from build123d import *

# Parameters (mm, degrees)
SKETCH_1_W          = 200
SKETCH_1_H          = 100
EXTRUDE_1_DEPTH     = 8
SKETCH_2_OUTSIDE_W  = 246.75
SKETCH_2_OUTSIDE_H  = 146.75
CUT_EXTRUDE_1_DEPTH = 223.081848133
SKETCH_3_R          = 2
SKETCH_3_R_2        = 4
CUT_EXTRUDE_2_DEPTH = 184.742611471


with BuildPart() as part:
    # 草图1 → 凸台-拉伸1 (new body)
    with BuildSketch(Plane.XY):
        with Locations((100, 46.209912536)):
            Rectangle(SKETCH_1_W, SKETCH_1_H)
    extrude(amount=EXTRUDE_1_DEPTH)

    # 草图2 outside → 切除-拉伸1 (cut, through all)
    with BuildSketch(Plane.XY.offset(8)):
        with Locations((100, 46.21)):
            Rectangle(SKETCH_2_OUTSIDE_W, SKETCH_2_OUTSIDE_H)
        with BuildLine():
            Line((156, 96.209912536), (156, 53.259476571))
            ThreePointArc((156, 53.259476571), (97.731456144, 1.942362699), (44, 57.992340397))
            Line((44, 57.992340397), (44, 96.209912536))
            Line((44, 96.209912536), (56, 96.209912536))
            Line((56, 96.209912536), (56, 57.992340397))
            ThreePointArc((56, 57.992340397), (98, 13.942368774), (144, 53.797105004))
            Line((144, 53.797105004), (144, 96.209912536))
            Line((144, 96.209912536), (156, 96.209912536))
        make_face(mode=Mode.SUBTRACT)
    extrude(amount=-CUT_EXTRUDE_1_DEPTH, mode=Mode.SUBTRACT)

    # 草图3 → 切除-拉伸2 (cut, through all)
    with BuildSketch(Plane.XY.offset(13)):
        with Locations((48.3, 87.392340397)):
            Circle(SKETCH_3_R)
        with Locations((56.8, 35.392340397)):
            Circle(SKETCH_3_R)
        with Locations((143.2, 35.392340397)):
            Circle(SKETCH_3_R)
        with Locations((151.7, 87.392340397)):
            Circle(SKETCH_3_R)
        with Locations((100, 7.692340397)):
            Circle(SKETCH_3_R_2)
    extrude(amount=-CUT_EXTRUDE_2_DEPTH, mode=Mode.SUBTRACT)


solid = part.part
Read the model definition and answer for the solid it produces. Units are mm, in the model's axes. A direction names the side the tool comes from. Round coordinates to 2 decimals unless told otherwise and drop trailing zeros. Write each loop counter-clockwise with the first axis right and the second up, starting at its lowest first coordinate (ties: lowest second). Pieces come first, ordered by that corner, then holes. Notation, with made-up numbers: (47, 56) - (105, 56) arc R15 ccw to (105, 78) - close; hole circle Ø11 at (47, -24.5). An arc over 180 degrees is marked (long way). Use a Markdown table: item, result.
(1) Each of these flat-tipped pins is pushed along its axis until it touches: pin 1 Ø3 at (y, z) = (35.5, 6.5) entering from +X; pin 2 Ø12 at (x, y) = (100, 25.5) entering from +Z; pin 3 Ø2 at (x, z) = (131.5, 3) entering from +Y; pin 4 Ø4 at (x, z) = (137, 1.5) entering from +Y. Where does it stop, or does it pass through?
Reported:
| item | result |
|---|---|
| pin 1 | x = 152.12 |
| pin 2 | through |
| pin 3 | y = 28.07 |
| pin 4 | y = 37.22 |
(2) The part is cut by section A-A (x = 100). Write down the section's boundary in (y, z).
Reported:
| item | result |
|---|---|
| outline | (1.89, 0) - (3.69, 0) - (3.69, 8) - (1.89, 8) - close; (11.69, 0) - (13.89, 0) - (13.89, 8) - (11.69, 8) - close |
(3) Straight lines are drawn through the part: line 1 along X through (y, z) = (84.5, 1); line 2 along X through (y, z) = (88, 1); line 3 along Y through (x, z) = (100, 4.75). For each, find the intervals that lie inside material, in ascending order. Write a range as [from, to].
Reported:
| item | result |
|---|---|
| line 1 | [44, 56], [144, 156] |
| line 2 | [44, 46.39], [50.21, 56], [144, 149.79], [153.61, 156] |
| line 3 | [1.89, 3.69], [11.69, 13.89] |
(4) The part is cut by section C-C (x = 48.3). Write down the section's boundary in (y, z), then the cut area to 3 significant figures.
Reported:
| item | result |
|---|---|
| outline | (36.45, 0) - (85.39, 0) - (85.39, 8) - (36.45, 8) - close; (89.39, 0) - (96.21, 0) - (96.21, 8) - (89.39, 8) - close |
| area | 446 mm2 |
(5) The mould has two halves that part along Y. Classify faces 3 (the flat face through (56, 77, 4)), 4 (the flat face through (150, 96.21, 4)), 5 (the cylindrical face through (145.11, 35.99, 4.06)): released by +Y, released by -Y, zero draft, split by the parting line, or undercut.
Reported:
| item | result |
|---|---|
| face 3 | zero draft |
| face 4 | released by +Y |
| face 5 | undercut |
(6) The part is cut by section D-D (x = 126). Write down the section's boundary in (y, z).
Reported:
| item | result |
|---|---|
| outline | (8.23, 0) - (22.3, 0) - (22.3, 8) - (8.23, 8) - close |
(7) The part is cut by section B-B (z = 2.5). Write down the section's boundary in (x, y).
Reported:
| item | result |
|---|---|
| outline | (44, 57.99) arc R56.1 ccw to (156, 53.26) - (156, 96.21) - (144, 96.21) - (144, 53.8) arc R44.1 cw to (56, 57.99) - (56, 96.21) - (44, 96.21) - close; hole circle Ø4 at (48.3, 87.39); hole circle Ø4 at (56.8, 35.39); hole circle Ø8 at (100, 7.69); hole circle Ø4 at (143.2, 35.39); hole circle Ø4 at (151.7, 87.39) |
(8) Which of the six approach directions +Z, -Z, +X, -X, +Y, -Y give full straight-line access (tool end or side, diameter ignored) to faces 1 (the cylindrical face through (98.931, 1.905, 4.056)), 2 (the flat face through (144, 75, 4))?
Reported:
| item | result |
|---|---|
| face 1 | +Z, -Z, -Y |
| face 2 | +Z, -Z, +Y |
